from build123d import *

# Parameters (mm, degrees)
BOSS_EXTRUDE1_DEPTH = 3.5
BOSS_EXTRUDE2_DEPTH = 21
SKETCH3_W           = 23
SKETCH3_H           = 39
BOSS_EXTRUDE3_DEPTH = 2.5
SKETCH5_W           = 21.5
SKETCH5_H           = 25
SKETCH5_W_2         = 7.07
SKETCH5_H_2         = 19.04
BOSS_EXTRUDE5_DEPTH = 2.5
SKETCH6_W           = 7.07
SKETCH6_H           = 5.9
BOSS_EXTRUDE6_DEPTH = 20
BOSS_EXTRUDE7_DEPTH = 23
FILLET1_SIZE        = 10
SKETCH9_R           = 2.475
BOSS_EXTRUDE8_DEPTH = 9
FILLET2_R           = 0.5
SKETCH10_R          = 1.65
CUT_EXTRUDE1_DEPTH  = 9
SKETCH11_W          = 0.2
SKETCH11_H          = 20
CUT_EXTRUDE2_DEPTH  = 9
CUT_EXTRUDE3_DEPTH  = 9
FILLET3_SIZE        = 3
BOSS_EXTRUDE9_DEPTH = 5
SKETCH14_R          = 1.747814763
SKETCH14_R_2        = 1.6
CUT_EXTRUDE4_DEPTH  = 15
CUT_EXTRUDE5_DEPTH  = 113
FILLET4_SIZE        = 7
FILLET5_SIZE        = 3
FILLET6_SIZE        = 3
FILLET7_R           = 1
SKETCH16_W          = 8
SKETCH16_H          = 21
CUT_EXTRUDE6_DEPTH  = 113
FILLET8_R           = 1


# Some blends are built 0.0001 mm under size
with BuildPart() as part:
    # Sketch1 → Boss-Extrude1 (new body)
    with BuildSketch(Plane(origin=(0, 0, 0), x_dir=(1, 0, 0), z_dir=(0, 1, 0))):
        Polygon((0, 40), (23, 40), (23, 79), (0, 79), (0, 100), (110, 100), (110, 79), (87, 79), (87, 40), (110, 40), (110, 20), (80, 0), (30, 0), (0, 20), align=None)
    extrude(amount=BOSS_EXTRUDE1_DEPTH)

    # Sketch2 → Boss-Extrude2 (add)
    with BuildSketch(Plane(origin=(0, 3.5, 0), x_dir=(1, 0, 0), z_dir=(0, 1, 0))):
        Polygon((0, 79), (23, 79), (23, 40), (0, 40), (0, 37.5), (25.5, 37.5), (25.5, 81.5), (0, 81.5), align=None)
        Polygon((110, 81.5), (84.5, 81.5), (84.5, 37.5), (110, 37.5), (110, 40), (87, 40), (87, 79), (110, 79), align=None)
    extrude(amount=BOSS_EXTRUDE2_DEPTH)

    # Sketch3 → Boss-Extrude3 (add)
    with BuildSketch(Plane(origin=(0, 24.5, 0), x_dir=(1, 0, 0), z_dir=(0, 1, 0))):
        with Locations((11.5, 59.5)):
            Rectangle(SKETCH3_W, SKETCH3_H)
        with Locations((98.5, 59.5)):
            Rectangle(SKETCH3_W, SKETCH3_H)
    extrude(amount=-BOSS_EXTRUDE3_DEPTH)

    # Sketch5 → Boss-Extrude5 (add)
    with BuildSketch(Plane(origin=(0, 24.5, 0), x_dir=(1, 0, 0), z_dir=(0, 1, 0))):
        with Locations((120.75, 50)):
            Rectangle(SKETCH5_W, SKETCH5_H)
        with Locations((-10.75, 50)):
            Rectangle(SKETCH5_W, SKETCH5_H)
        with Locations((29.035, 47.02)):
            Rectangle(SKETCH5_W_2, SKETCH5_H_2)
        with Locations((80.965, 47.02)):
            Rectangle(SKETCH5_W_2, SKETCH5_H_2)
    extrude(amount=-BOSS_EXTRUDE5_DEPTH)

    # Sketch6 → Boss-Extrude6 (add)
    with BuildSketch(Plane(origin=(0, 24.5, 0), x_dir=(1, 0, 0), z_dir=(0, 1, 0))):
        with Locations((29.035, 53.59)):
            Rectangle(SKETCH6_W, SKETCH6_H)
        with Locations((80.965, 53.59)):
            Rectangle(SKETCH6_W, SKETCH6_H)
        with Locations((-17.965, 53.59)):
            Rectangle(SKETCH6_W, SKETCH6_H)
        with Locations((127.965, 53.59)):
            Rectangle(SKETCH6_W, SKETCH6_H)
    extrude(amount=BOSS_EXTRUDE6_DEPTH)

    # Sketch7 → Boss-Extrude7 (add)
    with BuildSketch(Plane(origin=(0, 24.5, 0), x_dir=(1, 0, 0), z_dir=(0, 1, 0))):
        Polygon((0, 81.5), (25.5, 81.5), (25.5, 79), (0, 79), (-21.5, 79), (-21.5, 81.5), align=None)
        Polygon((110, 79), (84.5, 79), (84.5, 81.5), (110, 81.5), (131.5, 81.5), (131.5, 79), align=None)
    extrude(amount=BOSS_EXTRUDE7_DEPTH)

    # Fillet1
    # the kernel refuses this chamfer: 10 mm, written as the material it adds along each edge
    with BuildSketch(Plane(origin=(0, 22, -40), x_dir=(0.027495876610586372, -0.9996219169112968, 0), z_dir=(0, 0, 1)), Plane(origin=(110, 22, -37.5), x_dir=(-0.027495876610586317, -0.9996219169112968, 0), z_dir=(0, 0, -1)), Plane(origin=(110, 24.5, -81.5), x_dir=(0.9996219169112968, 0.027495876610586317, 0), z_dir=(0, 0, 1))) as fillet1_piece_1:
        Polygon((FILLET1_SIZE * 0.999621916911, -FILLET1_SIZE * 0.0274958766106), (-FILLET1_SIZE * 0.0274958766106, -FILLET1_SIZE * 0.999621916911), (0, 0), align=None)
    extrude(amount=2.5)
    with BuildSketch(Plane(origin=(0, 24.5, -79), x_dir=(0.027495876610586372, -0.9996219169112968, 0), z_dir=(0, 0, -1))) as fillet1_piece_2:
        Polygon((FILLET1_SIZE * 0.999621916911, FILLET1_SIZE * 0.0274958766106), (-FILLET1_SIZE * 0.0274958766106, FILLET1_SIZE * 0.999621916911), (0, 0), align=None)
    extrude(amount=2.5)

    # Sketch9 → Boss-Extrude8 (add)
    with BuildSketch(Plane(origin=(0, 0, -81.5), x_dir=(-1, 0, 0), z_dir=(0, 0, -1))):
        with Locations(Location((-114.55, 34.35, 0), (0, 0, 180))):
            Circle(SKETCH9_R)
        with Locations(Location((4.55, 34.35, 0), (0, 0, 180))):
            Circle(SKETCH9_R)
    extrude(amount=BOSS_EXTRUDE8_DEPTH)

    # Fillet2
    fillet2_edges = [part.edges().sort_by_distance(p)[0] for p in [
        (112.075, 34.35, -90.5),
        (-7.025, 34.35, -90.5),
    ]]
    fillet(fillet2_edges, radius=FILLET2_R)

    # Sketch10 → Cut-Extrude1 (cut)
    with BuildSketch(Plane.XY.offset(-50.64)):
        with Locations((129.16, 39.27)):
            Circle(SKETCH10_R)
        with Locations((129.16, 29.43)):
            Circle(SKETCH10_R)
        with Locations((79.77, 39.27)):
            Circle(SKETCH10_R)
        with Locations((79.77, 29.43)):
            Circle(SKETCH10_R)
        with Locations((-19.16, 29.43)):
            Circle(SKETCH10_R)
        with Locations((-19.16, 39.27)):
            Circle(SKETCH10_R)
        with Locations(Location((30.23, 39.27, 0), (0, 0, 180))):
            Circle(SKETCH10_R)
        with Locations(Location((30.23, 29.43, 0), (0, 0, 180))):
            Circle(SKETCH10_R)
    extrude(amount=-CUT_EXTRUDE1_DEPTH, mode=Mode.SUBTRACT)

    # Sketch11 → Cut-Extrude2 (cut)
    with BuildSketch(Plane.XY.offset(-50.64)):
        with Locations((-14.53, 34.5)):
            Rectangle(SKETCH11_W, SKETCH11_H)
        with Locations((25.6, 34.5)):
            Rectangle(SKETCH11_W, SKETCH11_H)
        with Locations((84.4, 34.5)):
            Rectangle(SKETCH11_W, SKETCH11_H)
        with Locations((124.53, 34.5)):
            Rectangle(SKETCH11_W, SKETCH11_H)
    extrude(amount=-CUT_EXTRUDE2_DEPTH, mode=Mode.SUBTRACT)

    # Sketch12 → Cut-Extrude3 (cut)
    with BuildSketch(Plane(origin=(0, 0, -81.5), x_dir=(-1, 0, 0), z_dir=(0, 0, -1))):
        Polygon((-108, 47.5), (-84.5, 25.5), (-84.5, 47.5), align=None)
        Polygon((-25.5, 25.5), (-25.5, 47.5), (-2, 47.5), align=None)
        Polygon((-120, 24.5), (-131.5, 36), (-131.5, 24.5), align=None)
        Polygon((10, 24.5), (21.5, 36), (21.5, 24.5), align=None)
    extrude(amount=-CUT_EXTRUDE3_DEPTH, mode=Mode.SUBTRACT)

    # Fillet3
    fillet3_edges = [part.edges().sort_by_distance(p)[0] for p in [
        (0, 23.25, -62.5),
        (110, 23.25, -62.5),
    ]]
    chamfer(fillet3_edges, length=FILLET3_SIZE)

    # Sketch13 → Boss-Extrude9 (add)
    with BuildSketch(Plane(origin=(0, 3.5, 0), x_dir=(1, 0, 0), z_dir=(0, 1, 0))):
        Polygon((0, 30.5), (32.5, 30.5), (32.5, 88.5), (0, 88.5), (0, 81.5), (25.5, 81.5), (25.5, 37.5), (0, 37.5), align=None)
        Polygon((84.5, 37.5), (110, 37.5), (110, 30.5), (77.5, 30.5), (77.5, 88.5), (110, 88.5), (110, 81.5), (84.5, 81.5), align=None)
    extrude(amount=BOSS_EXTRUDE9_DEPTH)

    # Sketch14 → Cut-Extrude4 (cut)
    with BuildSketch(Plane(origin=(0, 8.5, 0), x_dir=(1, 0, 0), z_dir=(0, 1, 0))):
        with Locations(Location((7.25, 34, 0), (0, 0, 270))):
            Circle(SKETCH14_R)
        with Locations(Location((7.25, 85, 0), (0, 0, 270))):
            Circle(SKETCH14_R_2)
        with Locations(Location((29, 34, 0), (0, 0, 270))):
            Circle(SKETCH14_R_2)
        with Locations(Location((29, 59.5, 0), (0, 0, 270))):
            Circle(SKETCH14_R_2)
        with Locations(Location((29, 85, 0), (0, 0, 270))):
            Circle(SKETCH14_R_2)
        with Locations(Location((81, 34, 0), (0, 0, 90))):
            Circle(SKETCH14_R_2)
        with Locations(Location((102.75, 34, 0), (0, 0, 90))):
            Circle(SKETCH14_R)
        with Locations(Location((81, 59.5, 0), (0, 0, 90))):
            Circle(SKETCH14_R_2)
        with Locations(Location((81, 85, 0), (0, 0, 90))):
            Circle(SKETCH14_R_2)
        with Locations(Location((102.75, 85, 0), (0, 0, 90))):
            Circle(SKETCH14_R_2)
    extrude(amount=-CUT_EXTRUDE4_DEPTH, mode=Mode.SUBTRACT)

    # Sketch15 → Cut-Extrude5 (cut)
    with BuildSketch(Plane(origin=(0, 0, -100), x_dir=(-1, 0, 0), z_dir=(0, 0, -1))):
        Polygon((-110, 3.5), (-32.5, 3.5), (-32.5, 47.5), (-131.5, 47.5), (-131.5, 3.5), align=None)
        Polygon((0, 0), (0, 3.5), (-32.5, 3.5), (-110, 3.5), (-110, 0), align=None)
    extrude(amount=-CUT_EXTRUDE5_DEPTH, mode=Mode.SUBTRACT)

    # Fillet4
    fillet4_edges = [part.edges().sort_by_distance(p)[0] for p in [
        (25.5, 22, -47.02),
    ]]
    chamfer(fillet4_edges, length=FILLET4_SIZE - 0.0001)  # a hair under: the kernel refuses the full size

    # Fillet5
    fillet5_edges = [part.edges().sort_by_distance(p)[0] for p in [
        (23, 12.75, -40),
        (23, 12.75, -79),
        (23, 22, -59.5),
        (6.5, 22, -40),
        (11.5, 22, -79),
    ]]
    chamfer(fillet5_edges, length=FILLET5_SIZE)

    # Fillet6
    fillet6_edges = [part.edges().sort_by_distance(p)[0] for p in [
        (0, 21.75, -79),
    ]]
    chamfer(fillet6_edges, length=FILLET6_SIZE)

    # Fillet7
    fillet7_edges = [part.edges().sort_by_distance(p)[0] for p in [
        (0, 6, -30.5),
        (32.5, 6, -30.5),
        (32.5, 6, -88.5),
        (0, 6, -88.5),
    ]]
    fillet(fillet7_edges, radius=FILLET7_R)

    # Sketch16 → Cut-Extrude6 (cut)
    with BuildSketch(Plane.XZ.offset(-22)):
        with Locations((10, -59.5)):
            Rectangle(SKETCH16_W, SKETCH16_H)
    extrude(amount=-CUT_EXTRUDE6_DEPTH, mode=Mode.SUBTRACT)

    # Fillet8
    fillet8_edges = [part.edges().sort_by_distance(p)[0] for p in [
        (6, 23.25, -70),
        (6, 23.25, -49),
        (14, 23.25, -49),
        (14, 23.25, -70),
    ]]
    fillet(fillet8_edges, radius=FILLET8_R)


solid = part.part
The listing builds one solid part. Answer for the finished solid, in the listing's coordinates (mm). A direction names the side the tool comes from. Round coordinates to 2 decimals unless told otherwise and drop trailing zeros. Order: outer loops, then holes, each group sorted by start corner. A loop starts at its lowest first (then second) coordinate and runs counter-clockwise, first axis right, second up. Notation, with made-up numbers: (-21.75, 78.25) - (3.25, 78.25) arc R34 ccw to (3.25, 111.25) - close; hole circle Ø4 at (-10, 84). An arc over 180 degrees is marked (long way). Write item = value, one per line. Start each with the question number.
1) Section A-A, the plane z = -85 is taken. Write down the section's boundary in (x, y) (3 decimals), plus the area to 3 significant figures.
2) Straight lines are drawn through the part: L1, parallel to Y at x = -19.16, z = -54.85; L2, parallel to X at y = 5.35, z = -34; L3, parallel to Z at x = 8.5, y = 18. For each, find the intervals that lie inside material, in ascending order.
3) Section C-C, the plane z = -34 is taken. Write down the section's boundary in (x, y), plus the area to 3 significant figures.
4) Given pin 1 (2.5 mm diameter, centred on x = 20, y = 6, fed in from -Z); pin 2 (4.5 mm diameter, centred on x = 7.25, z = -34, fed in from +Y); pin 3 (6 mm diameter, centred on x = 8.5, z = -53, fed in from -Y); pin 4 (5 mm diameter, centred on x = 7.25, z = -85, fed in from -Y), each flat-ended and moving along its own axis, determine where each tip first touches the part or whether it passes through.
5) For a pull along Z with two mould halves and no side action, classify faces 1 (the flat face through (2, 26, -79)), 2 (the flat face through (0, 7, -37)), 3 (the flat face through (-5, 34, -90.5)) as released by +Z, released by -Z, zero draft, split by the parting line, or undercut.
6) Section D-D, the plane y = 29.43 is taken. Write down the section's boundary in (x, z).
7) For faces 4 (the flat face through (-18, 34, -50.64)), 5 (the flat face through (26, 8.5, -57)), 6 (the flat face through (14, 23, -60)), 7 (the flat face through (-12, 23, -62.5)), 8 (the flat face through (5, 21, -42)), determine the directions among +Z, -Z, +X, -X, +Y, -Y from which every point of the face is accessible in a straight line to the end or side of a thin tool.
8) Section B-B, the plane x = -4.55 is taken. Write down the section's boundary in (y, z) (3 decimals), plus the area to 3 significant figures.
Results list:
q1.outline = circle Ø4.95 at (-4.55, 34.35); (0, 3.5) - (5.65, 3.5) - (5.65, 8.5) - (0, 8.5) - close; (8.85, 3.5) - (27.4, 3.5) - (27.4, 8.5) - (8.85, 8.5) - close; (30.6, 3.5) - (32.5, 3.5) - (32.5, 8.5) - (30.6, 8.5) - close
q1.area = 150 mm^2
q2.L1 = 22 to 27.78, 31.08 to 37.62, 40.92 to 44.5
q2.L2 = 0 to 5.5, 9 to 27.4, 30.6 to 32.5
q2.L3 = -81.5 to -79, -40 to -37.5
q3.outline = (0, 3.5) - (5.5, 3.5) - (5.5, 8.5) - (0, 8.5) - close; (9, 3.5) - (27.4, 3.5) - (27.4, 8.5) - (9, 8.5) - close; (30.6, 3.5) - (32.5, 3.5) - (32.5, 8.5) - (30.6, 8.5) - close
q3.area = 129 mm^2
q4.pin_1 = -88.5
q4.pin_2 = 8.5
q4.pin_3 = 22
q4.pin_4 = 3.5
q5.face_1 = undercut
q5.face_2 = zero draft
q5.face_3 = released by -Z
q6.outline = (-21.5, -56.54) - (-20.81, -56.54) - (-20.81, -50.64) - (-21.5, -50.64) - close; (-17.51, -56.54) - (-14.63, -56.54) - (-14.63, -50.64) - (-17.51, -50.64) - close; (-14.93, -81.5) - (21.3, -81.5) - (21.3, -79) - (-14.93, -79) - close; (25.7, -56.54) - (28.58, -56.54) - (28.58, -50.64) - (25.7, -50.64) - close; (31.88, -56.54) - (32.5, -56.54) - (32.5, -50.64) - (31.88, -50.64) - close
q7.face_4 = +Z, +X, -X, +Y
q7.face_5 = +X
q7.face_6 = +Y, -Y
q7.face_7 = -X, +Y, -Y
q7.face_8 = -X, -Y
q8.outline = (16.55, -40) - (19, -40) - (22, -43) - (22, -62.5) - (24.5, -62.5) - (24.5, -37.5) - (16.55, -37.5) - close; (19.05, -81.5) - (31.875, -81.5) - (31.875, -90) arc R0.5 ccw to (32.375, -90.5) - (36.325, -90.5) arc R0.5 ccw to (36.825, -90) - (36.825, -81.5) - (47.5, -81.5) - (47.5, -79) - (19.05, -79) - close
q8.area = 196 mm^2
